Answer from the drawing. Dimensions are ordinates in mm from the lowest x, y and z of the part. Round coordinates to 2 decimals unless told otherwise and drop trailing zeros. Loops run counter-clockwise (first coordinate to the right, second up) from the corner with the lowest first, then second, coordinate; pieces in that order, holes last. Notation, with made-up numbers: M 29.25,64 L 57.25,64 A14 cw 57.25,74 Z; hole C 49,10 d1. An arc over 180 degrees is marked long. Write each question's results on one line, items separated by ' | '.
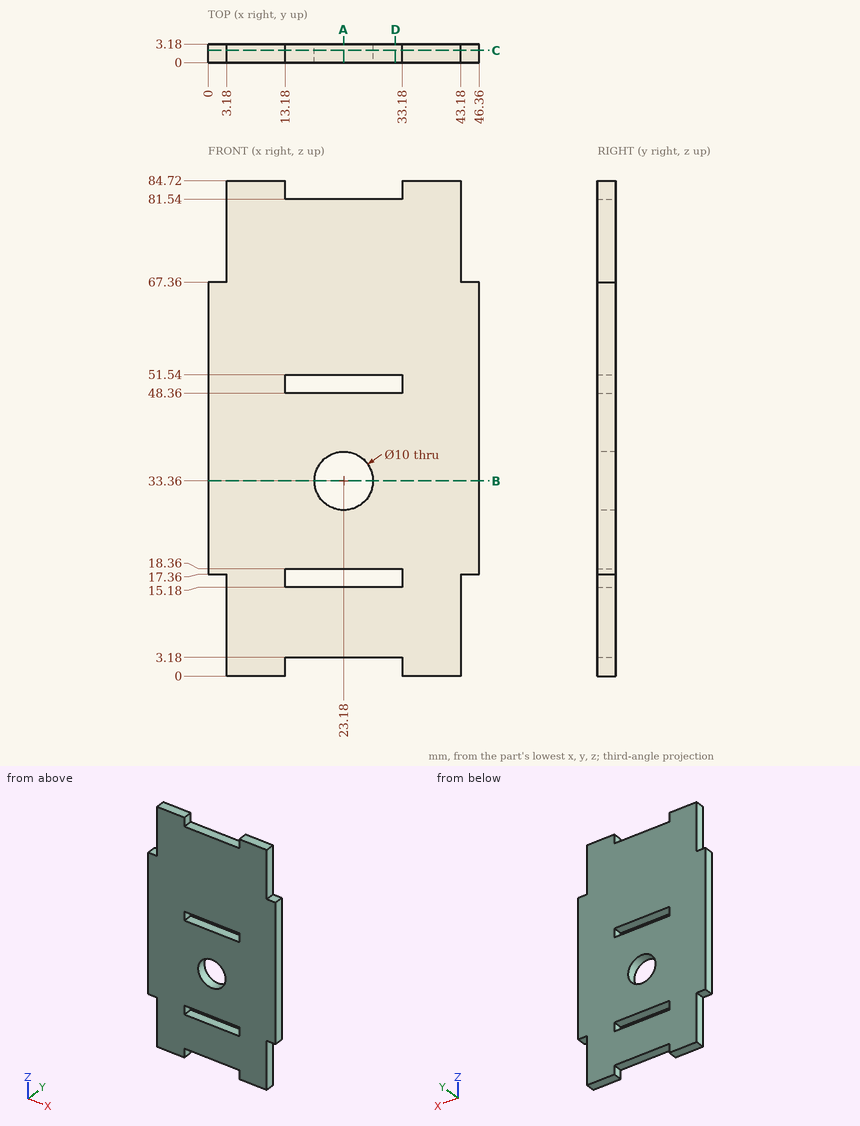
1. Find section D-D, the plane x = 32. Give the vertices of the cut face in (y, z), then the cut area to 3 significant figures.
Completed:
outline: M 0,3.18 L 3.18,3.18 L 3.18,15.18 L 0,15.18 Z; M 0,18.36 L 3.18,18.36 L 3.18,48.36 L 0,48.36 Z; M 0,51.54 L 3.18,51.54 L 3.18,81.54 L 0,81.54 Z | area: 229 mm2
2. Find section C-C, the plane y = 2.1. Count the separate pieces of the cut face and the enclosed holes in it, then the cut area to 3 significant figures.
Completed:
separate pieces: 1 | enclosed holes: 3 | area: 3,370 mm2
3. Given P1, Ø1, axis at x = 20, y = 2, coming from the -Z side; P2, Ø1, axis at x = 2, y = 1.5, coming from the +Z side; P3, Ø1, axis at x = 1, y = 1, coming from the -Z side; P4, Ø8, axis at x = 23.18, z = 33.36, coming from the +Y side, each flat-ended and moving along its own axis, determine where each tip first touches the part or whether it passes through.
Completed:
P1: stops at z = 3.18 | P2: stops at z = 67.36 | P3: stops at z = 17.36 | P4: passes through
4. Find the intervals of material crossed by L1, parallel to Z at x = 23.18, y = 1.95; L2, parallel to Z at x = 16, y = 3.05; L3, parallel to X at y = 2.4, z = 51, in increasing order.
Completed:
L1: z = 3.18 to 15.18, 18.36 to 28.36, 38.36 to 48.36, 51.54 to 81.54 | L2: z = 3.18 to 15.18, 18.36 to 48.36, 51.54 to 81.54 | L3: x = 0 to 13.18, 33.18 to 46.36
5. Find section B-B, the plane z = 33.36. Give the vertices of the cut face in (x, y), then the cut area to 3 significant figures.
Completed:
outline: M 0,0 L 18.18,0 L 18.18,3.18 L 0,3.18 Z; M 28.18,0 L 46.36,0 L 46.36,3.18 L 28.18,3.18 Z | area: 116 mm2
6. Find section A-A, the plane x = 23.18. Give the vertices of the cut face in (y, z), then the cut area to 3 significant figures.
Completed:
outline: M 0,3.18 L 3.18,3.18 L 3.18,15.18 L 0,15.18 Z; M 0,18.36 L 3.18,18.36 L 3.18,28.36 L 0,28.36 Z; M 0,38.36 L 3.18,38.36 L 3.18,48.36 L 0,48.36 Z; M 0,51.54 L 3.18,51.54 L 3.18,81.54 L 0,81.54 Z | area: 197 mm2
